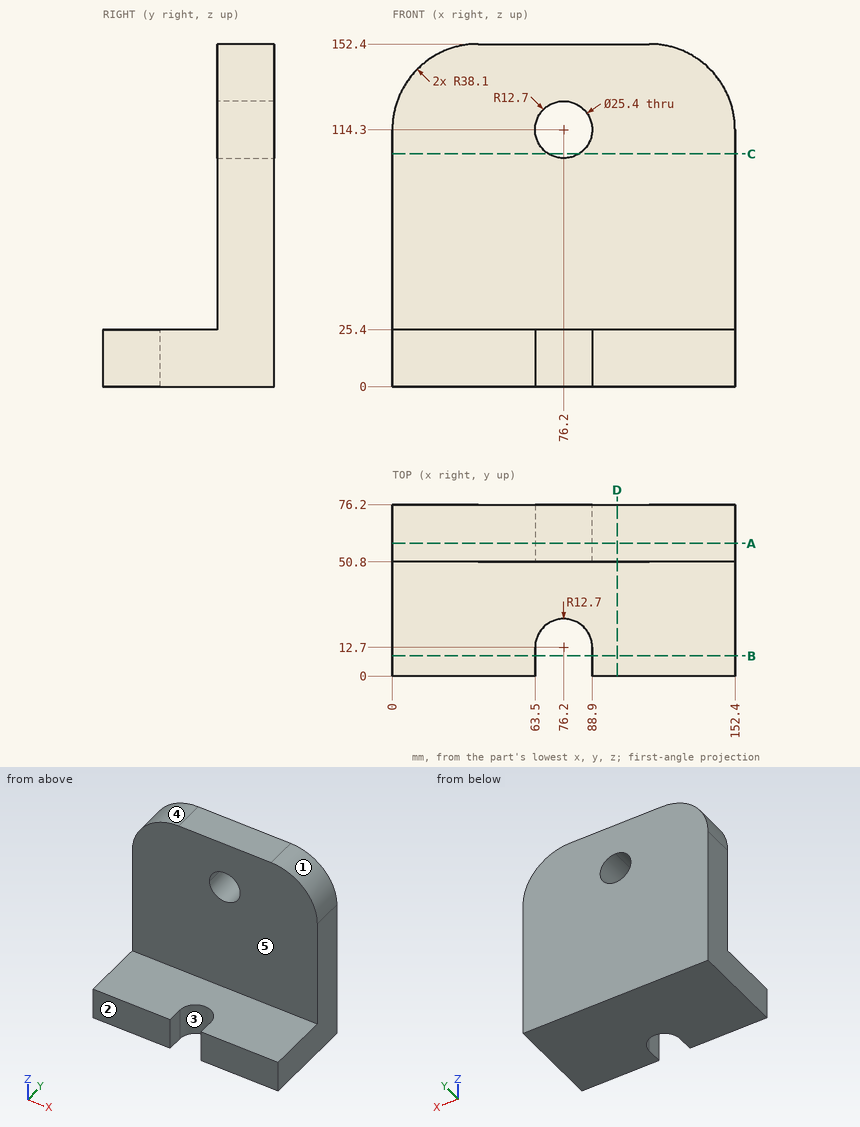
For this review, use the dimensioned drawing (mm, ordinates from the lowest corner) and the shaded views. A direction names the side the tool comes from. Round coordinates to 2 decimals unless told otherwise and drop trailing zeros. Write each loop counter-clockwise with the first axis right and the second up, starting at its lowest first coordinate (ties: lowest second). Pieces come first, ordered by that corner, then holes. Notation, with made-up numbers: (-16, 63.25) - (0, 63.25) arc R23 cw to (0, 84.25) - close; hole circle Ø4 at (26.25, -7.5). An arc over 180 degrees is marked (long way). Answer as a JSON object with one key per item and string values.
1. Tool access review of the marked faces 4 and 5: name each direction out of +Z, -Z, +X, -X, +Y, -Y from which nothing blocks a thin tool from reaching the whole face with its end or side.
Response values:
{"face 4": "+Z, -X, +Y, -Y", "face 5": "+Z, +X, -X, -Y"}
2. We need section B-B on y = 9. Give the boundary of the cut face in (x, z), then the cut area to 3 significant figures.
Response values:
{"outline": "(0, 0) - (63.5, 0) - (63.5, 25.4) - (0, 25.4) - close; (88.9, 0) - (152.4, 0) - (152.4, 25.4) - (88.9, 25.4) - close", "area": "3,230 mm2"}
3. We need section D-D on x = 100. Give the boundary of the cut face in (y, z).
Response values:
{"outline": "(0, 0) - (76.2, 0) - (76.2, 152.4) - (50.8, 152.4) - (50.8, 25.4) - (0, 25.4) - close"}
4. To check wall thickness, follow line 1 along X through (y, z) = (70, 114); line 2 along Z through (x, y) = (76, 58); line 3 along Z through (x, y) = (79, 49.5). State the ranges of each line that lie inside material, in increasing order.
Response values:
{"line 1": "x = 0 to 63.5, 88.9 to 152.4", "line 2": "z = 0 to 101.6, 127 to 152.4", "line 3": "z = 0 to 25.4"}
5. For pin 1 Ø12 at (x, z) = (115.5, 117) entering from -Y; pin 2 Ø4 at (y, z) = (66.5, 135) entering from -X; pin 3 Ø23 at (x, z) = (76.2, 114.3) entering from +Y, all flat-tipped, find the tip position at first contact; note any pin that passes through.
Response values:
{"pin 1": "stops at y = 50.8", "pin 2": "stops at x = 4.9", "pin 3": "passes through"}
6. We need section C-C on z = 103.5. Give the boundary of the cut face in (x, y), then the cut area to 3 significant figures.
Response values:
{"outline": "(0, 50.8) - (69.52, 50.8) - (69.52, 76.2) - (0, 76.2) - close; (82.88, 50.8) - (152.4, 50.8) - (152.4, 76.2) - (82.88, 76.2) - close", "area": "3,530 mm2"}
7. We need section A-A on y = 59. Give the boundary of the cut face in (x, z).
Response values:
{"outline": "(0, 0) - (152.4, 0) - (152.4, 114.3) arc R38.1 ccw to (114.3, 152.4) - (38.1, 152.4) arc R38.1 ccw to (0, 114.3) - close; hole circle Ø25.4 at (76.2, 114.3)"}
8. Draft analysis for pull direction X (two halves, no side actions). For the marked faces 1, 2 and 3, state which applies: +X half, -X half, draft (parallel to the pull), parting line (faces both ways), or undercut.
Response values:
{"face 1": "+X half", "face 2": "draft", "face 3": "undercut"}
